Geometry check sheet. Reference: drawing and pictorial views, mm from the part's lowest x, y, z. A direction names the side the tool comes from. Give positions to 0.01 mm unless a question says otherwise; leave off trailing zeros. Write each loop counter-clockwise with the first axis right and the second up, starting at its lowest first coordinate (ties: lowest second). Pieces come first, ordered by that corner, then holes. Notation, with made-up numbers: M 26.5,60 L 58.5,60 A17 ccw 58.5,92 Z; hole C 7.5,52 d6. An arc over 180 degrees is marked long. One line per item, written item: value. Start each with the question number.
1. Tool access check on the marked faces 3 and 4. Record the directions out of +Z, -Z, +X, -X, +Y, -Y that give a thin tool (end or side, any length) a straight path to the whole face; none if there is none.
2. Cross-section at D-D on x = 50. Record the cut outline in (y, z).
3. Cross-section at A-A on x = 33. Record the cut outline in (y, z) (1 decimal), then the cut area to 3 significant figures.
4. Scan lines: line 1 (X direction, y = 11.5, z = 28) (1 decimal); line 2 (Z direction, x = 28.5, y = 17.25); line 3 (Z direction, x = 20.5, y = 10.75) (1 decimal). Record each from-to range of solid material in increasing order.
5. Release check for a two-part mould opening along X. For the marked faces 1 and 2 record: pulls with the +X half, pulls with the -X half, needs draft (parallel to the pull), parting line crosses it, or undercut.
6. Gauge pin test, flat ends, axial feed: pin 1 (4.5 mm diameter, centred on x = 44.5, y = 14.5, fed in from +Z) (1 decimal); pin 2 (4.5 mm diameter, centred on x = 45.5, y = 13, fed in from -Z) (1 decimal); pin 3 (10 mm diameter, centred on y = 20.5, z = 21, fed in from -X). Record the tip position at first contact, or that the pin passes through.
7. Cross-section at B-B on z = 41. Record the cut outline in (x, y).
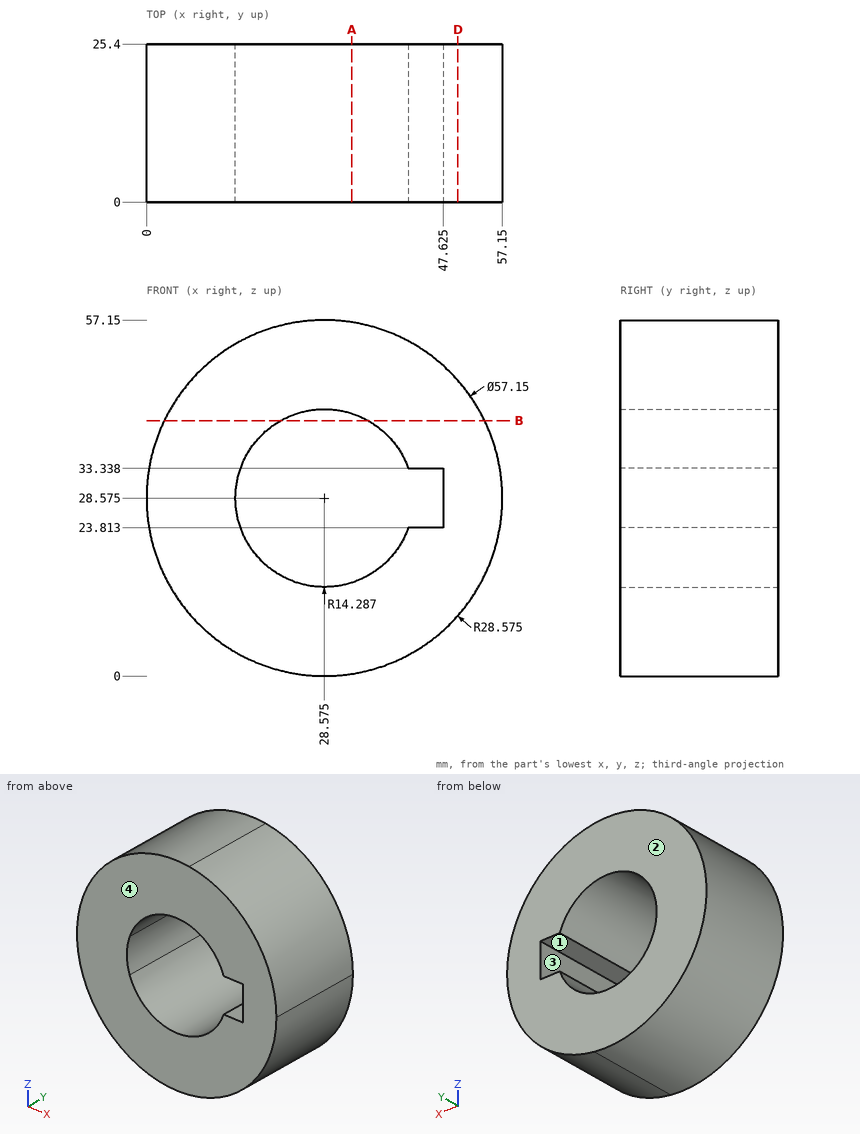
Report:
1. face 3: +Y, -Y
1. face 4: +Z, -Z, +X, -X, -Y
2. outline: M 0,9.67 L 25.4,9.67 L 25.4,47.48 L 0,47.48 Z
3. outline: M 0,0.3 L 25.4,0.3 L 25.4,15 L 0,15 Z; M 0,42.2 L 25.4,42.2 L 25.4,56.8 L 0,56.8 Z
3. area: 744 mm^2
4. line 1: x = 0 to 14.3, 47.6 to 57.1
4. line 2: z = 0 to 14.29, 42.86 to 57.15
4. line 3: z = 1.2 to 16.8, 40.4 to 56
5. face 1: undercut
5. face 2: needs draft
6. pin 1: stops at z = 53.7
6. pin 2: stops at z = 4.1
6. pin 3: stops at x = 0.12
7. outline: M 2.84,0 L 21.52,0 L 21.52,25.4 L 2.84,25.4 Z; M 35.63,0 L 54.31,0 L 54.31,25.4 L 35.63,25.4 Z
